The model under review builds one solid part; all positions refer to its coordinate system, in mm. A direction names the side the tool comes from. Coordinates: 2 decimals unless noted, no trailing zeros. Order: outer loops, then holes, each group sorted by start corner. A loop starts at its lowest first (then second) coordinate and runs counter-clockwise, first axis right, second up. Notation, with made-up numbers: M -12.5,-30 L 1.5,-30 A34 cw 1.5,9 Z; hole C 2.5,88.25 d2. An arc over 180 degrees is marked long. One line per item, written item: value.
```python
from build123d import *

# Parameters (mm, degrees)
ESQUISSE1_W             = 36.068
ESQUISSE1_H             = 48.26
BOSS_EXTRU_1_DEPTH      = 2
ESQUISSE4_R             = 3
BOSS_EXTRU_2_DEPTH      = 3
ESQUISSE6_R             = 1.5
ENL_V_MAT_EXTRU_1_DEPTH = 31.536569159
ESQUISSE10_W            = 48.26
ESQUISSE10_H            = 2
BOSS_EXTRU_3_DEPTH      = 3
ESQUISSE11_W            = 2.839594579
ESQUISSE11_H            = 48.26
BOSS_EXTRU_4_DEPTH      = 4.6
ESQUISSE12_W            = 48.26
ESQUISSE12_H            = 2.5
BOSS_EXTRU_5_DEPTH      = 5


with BuildPart() as part:
    # Esquisse1 → Boss.-Extru.1 (new body)
    with BuildSketch(Plane(origin=(0, 0, 0), x_dir=(1, 0, 0), z_dir=(0, 1, 0))):
        Rectangle(ESQUISSE1_W, ESQUISSE1_H)
    extrude(amount=BOSS_EXTRU_1_DEPTH)

    # Esquisse4 → Boss.-Extru.2 (add)
    with BuildSketch(Plane(origin=(0, 2, 0), x_dir=(1, 0, 0), z_dir=(0, 1, 0))):
        with Locations(Location((9.585669099, 18.921, 0), (0, 0, 270))):
            Circle(ESQUISSE4_R)
        with Locations(Location((9.585669099, -18.925, 0), (0, 0, 270))):
            Circle(ESQUISSE4_R)
    boss_extru_2 = extrude(amount=BOSS_EXTRU_2_DEPTH)

    # Esquisse6 → Enlèv. mat.-Extru.1 (cut, through all)
    with BuildSketch(Plane(origin=(0, 5, 0), x_dir=(1, 0, 0), z_dir=(0, 1, 0))):
        with Locations(Location((9.585669099, 18.921, 0), (0, 0, 270))):
            Circle(ESQUISSE6_R)
        with Locations(Location((9.585669099, -18.925, 0), (0, 0, 270))):
            Circle(ESQUISSE6_R)
    enl_v_mat_extru_1 = extrude(amount=-ENL_V_MAT_EXTRU_1_DEPTH, mode=Mode.SUBTRACT)

    # Symétrie1: Boss.-Extru.2, Enlèv. mat.-Extru.1 across plane
    add(boss_extru_2.mirror(Plane(origin=(0, 0, 0), x_dir=(0, 0, 1), z_dir=(1, 0, 0))))
    add(enl_v_mat_extru_1.mirror(Plane(origin=(0, 0, 0), x_dir=(0, 0, 1), z_dir=(1, 0, 0))), mode=Mode.SUBTRACT)

    # Esquisse10 → Boss.-Extru.3 (add)
    with BuildSketch(Plane(origin=(18.034, 0, 0), x_dir=(0, 0, -1), z_dir=(1, 0, 0))):
        with Locations((0, 1)):
            Rectangle(ESQUISSE10_W, ESQUISSE10_H)
    extrude(amount=BOSS_EXTRU_3_DEPTH)

    # Esquisse11 → Boss.-Extru.4 (add)
    with BuildSketch(Plane(origin=(0, 0, 0), x_dir=(-1, 0, 0), z_dir=(0, -1, 0))):
        with Locations((-19.614202711, 0)):
            Rectangle(ESQUISSE11_W, ESQUISSE11_H)
    extrude(amount=BOSS_EXTRU_4_DEPTH)

    # Esquisse12 → Boss.-Extru.5 (add)
    with BuildSketch(Plane.ZY.offset(-18.194405421)):
        with Locations((0, -3.35)):
            Rectangle(ESQUISSE12_W, ESQUISSE12_H)
    extrude(amount=BOSS_EXTRU_5_DEPTH)


solid = part.part
```
(1) We need section C-C, the plane x = -13.5. State the section outline as (y, z) points, plus the area to 3 significant figures.
Geometry results:
outline: M 0,-24.13 L 2,-24.13 L 2,24.13 L 0,24.13 Z
area: 96.5 mm2
(2) For L1, parallel to X at y = 1, z = 19; L2, parallel to Y at x = 15.5, z = -6.5; L3, parallel to X at y = -1.25, z = -5, list the stretches that pass through material, from the lowest coordinate up.
Geometry results:
L1: x = -18.03 to -11.08, -8.09 to 8.09, 11.08 to 21.03
L2: y = -4.6 to -2.1, 0 to 2
L3: x = 18.19 to 21.03
(3) Mouldability with a two-part tool opening along Z and no side actions: class faces 1 (the cylindrical face through (-9.718, 3.479, -21.918)), 2 (the flat face through (6, 1, 24.13)), 3 (the flat face through (-11, 5, 20)) as +Z half, -Z half, draft (parallel to the pull), parting line (faces both ways), or undercut.
Geometry results:
face 1: undercut
face 2: +Z half
face 3: draft
(4) We need section B-B, the plane z = -13.5. State the section outline as (x, y) points, plus the area to 3 significant figures.
Geometry results:
outline: M -18.03,0 L 18.19,0 L 18.19,-2.1 L 13.19,-2.1 L 13.19,-4.6 L 21.03,-4.6 L 21.03,2 L -18.03,2 Z
area: 104 mm2
(5) We need section A-A, the plane x = 16.5. State the section outline as (y, z) points, plus the area to 3 significant figures.
Geometry results:
outline: M -4.6,-24.13 L -2.1,-24.13 L -2.1,24.13 L -4.6,24.13 Z; M 0,-24.13 L 2,-24.13 L 2,24.13 L 0,24.13 Z
area: 217 mm2
(6) Tool access review of faces 4 (the cylindrical face through (9.718, 3.479, -21.918)), 5 (the flat face through (13.194, -3, 0)), 6 (the flat face through (18.194, -1, 0)), 7 (the flat face through (11, 5, -18)): name each direction out of +Z, -Z, +X, -X, +Y, -Y from which nothing blocks a thin tool from reaching the whole face with its end or side.
Geometry results:
face 4: +Y
face 5: +Z, -Z, -X, -Y
face 6: +Z, -Z, -X
face 7: +Z, -Z, +X, -X, +Y
(7) Insertion check: pin 1 Ø0.7 at (y, z) = (-3.5, 2.5) entering from -X; pin 2 Ø1.7 at (y, z) = (-1, -5) entering from -X; pin 3 Ø3.5 at (x, z) = (-9.59, -18.92) entering from +Y; pin 4 Ø4 at (x, z) = (-5, -15) entering from -Y. Each pin has a flat end and moves straight along its axis. Give the tip position at first contact, or say it passes through.
Geometry results:
pin 1: stops at x = 13.19
pin 2: stops at x = 18.19
pin 3: stops at y = 5
pin 4: stops at y = 0
(8) We need section D-D, the plane y = -3.5. State the section outline as (x, z) points, plus the area to 3 significant figures.
Geometry results:
outline: M 13.19,-24.13 L 21.03,-24.13 L 21.03,24.13 L 13.19,24.13 Z
area: 378 mm2
